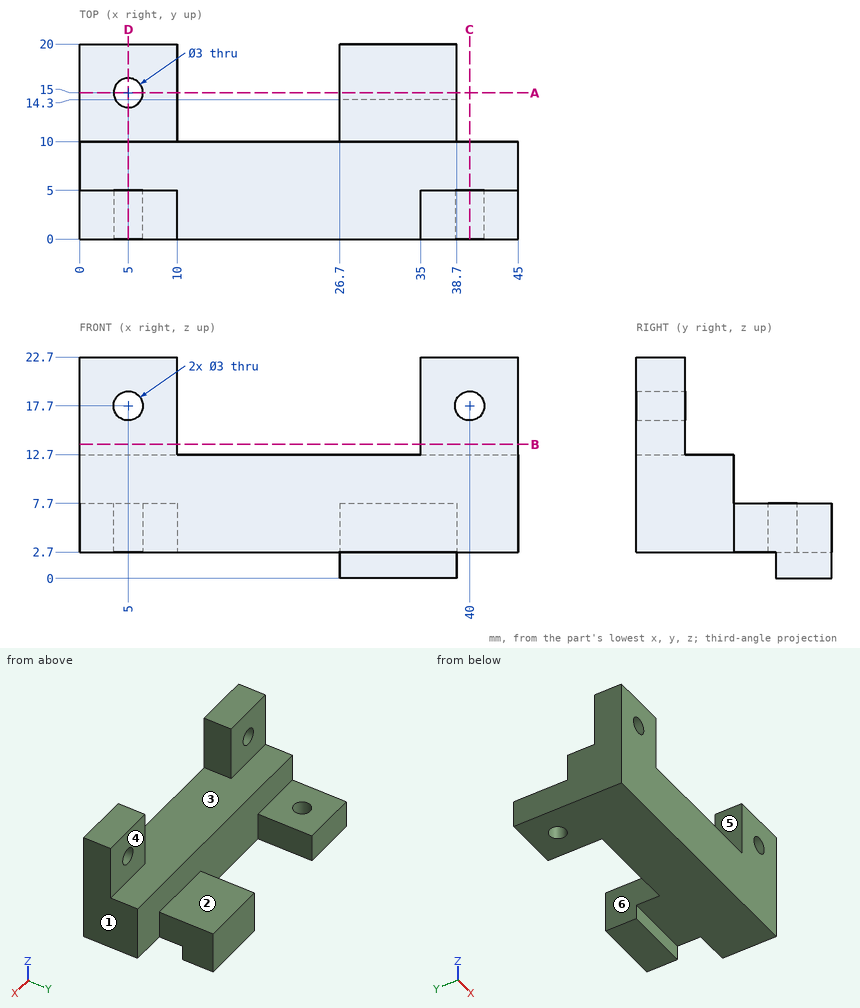
Geometry: see drawing. Coordinates: mm, zero at the bounding-box minimum. A direction names the side the tool comes from. Round coordinates to 2 decimals unless told otherwise and drop trailing zeros. Loops run counter-clockwise (first coordinate to the right, second up) from the corner with the lowest first, then second, coordinate; pieces in that order, holes last. Notation, with made-up numbers: M 12,69 L 60,69 A12 ccw 60,86 Z; hole C 16.5,85.5 d2. An arc over 180 degrees is marked long. Use a Markdown table: item, result. Add a question column.
1. Section query A-A on y = 15. Return the cut outline in (x, z), then the cut area to 3 significant figures.
2. Reachability of the marked faces 4, 5 and 6 from +Z, -Z, +X, -X, +Y, -Y: full face, straight path, thin tool, end or side. Return the list, or none.
3. Section query B-B on z = 13.75. Return the cut outline in (x, y), then the cut area to 3 significant figures.
4. Contact query for flat-ended pins moving along their axis: P1, Ø8, axis at x = 17, y = 3.5, coming from the +Z side; P2, Ø3.5, axis at x = 5, z = 17.7, coming from the +Y side; P3, Ø10, axis at y = 11.5, z = 4.5, coming from the -X side; P4, Ø3, axis at x = 4.5, y = 15.5, coming from the +Z side. Output: stop coordinate, or through.
5. Mould query, pull axis X, two halves, no side actions, for the marked faces 1, 2 and 3. Classes: pulls with the +X half, pulls with the -X half, needs draft (parallel to the pull), parting line crosses it, or undercut.
6. Section query D-D on x = 5. Return the cut outline in (y, z), then the cut area to 3 significant figures.
7. Section query C-C on x = 40. Return the cut outline in (y, z), then the cut area to 3 significant figures.
8. Line query: line 1 (Z direction, x = 40, y = 2.5); line 2 (Y direction, x = 5, z = 5.7); line 3 (X direction, y = 12.25, z = 3). Output: solid intervals per line, ascending.
Reported:
| question | item | result |
|---|---|---|
| 1 | outline | M 0,2.7 L 3.5,2.7 L 3.5,7.7 L 0,7.7 Z; M 6.5,2.7 L 10,2.7 L 10,7.7 L 6.5,7.7 Z; M 26.7,0 L 38.7,0 L 38.7,7.7 L 26.7,7.7 Z |
| 1 | area | 127 mm² |
| 2 | face 4 | +Z, +X, -X, +Y |
| 2 | face 5 | +Z, +Y, -Y |
| 2 | face 6 | +Z, -Z, +Y |
| 3 | outline | M 0,0 L 10,0 L 10,5 L 0,5 Z; M 35,0 L 45,0 L 45,5 L 35,5 Z |
| 3 | area | 100 mm² |
| 4 | P1 | stops at z = 12.7 |
| 4 | P2 | stops at y = 5 |
| 4 | P3 | stops at x = 0 |
| 4 | P4 | stops at z = 7.7 |
| 5 | face 1 | pulls with the +X half |
| 5 | face 2 | needs draft |
| 5 | face 3 | undercut |
| 6 | outline | M 0,2.7 L 13.5,2.7 L 13.5,7.7 L 10,7.7 L 10,12.7 L 5,12.7 L 5,16.2 L 0,16.2 Z; M 0,19.2 L 5,19.2 L 5,22.7 L 0,22.7 Z; M 16.5,2.7 L 20,2.7 L 20,7.7 L 16.5,7.7 Z |
| 6 | area | 170 mm² |
| 7 | outline | M 0,2.7 L 10,2.7 L 10,12.7 L 5,12.7 L 5,16.2 L 0,16.2 Z; M 0,19.2 L 5,19.2 L 5,22.7 L 0,22.7 Z |
| 7 | area | 135 mm² |
| 8 | line 1 | z = 2.7 to 16.2, 19.2 to 22.7 |
| 8 | line 2 | y = 0 to 13.5, 16.5 to 20 |
| 8 | line 3 | x = 0 to 10, 26.7 to 38.7 |
